Autodesk Inventor part; units mm, degrees
ref_plane "YZ Plane" through (0, 0, 0) normal (1, 0, 0) x (0, 1, 0)
ref_plane "XZ Plane" through (0, 0, 0) normal (0, 1, 0) x (-1, 0, 0)
ref_plane "XY Plane" through (0, 0, 0) normal (0, 0, 1) x (1, 0, 0)
sketch "Sketch1" plane through (0, 0, 0) normal (0, 0, 1) x (1, 0, 0)
  line L0 (0, 0) -> (15.24, 0)
  line L1 (15.24, 0) -> (15.24, 25.4)
  line L2 (15.24, 25.4) -> (0, 25.4)
  line L3 (0, 25.4) -> (0, 0)
  dimension "d0" = 15.24
  dimension "d1" = 25.4
extrude "Extrusion1" add sketch "Sketch1" along normal blind 3.175
sketch "Sketch2" plane through (0, 0, 3.175) normal (0, 0, 1) x (1, 0, 0)
  line L0 (15.24, 25.4) -> (0, 25.4)
  line L1 (0, 25.4) -> (4.826, 25.4)
  line L2 (4.826, 25.4) -> (4.826, 22.86)
  line L3 (4.826, 22.86) -> (0, 22.86)
  line L4 (0, 22.86) -> (0, 25.4)
  line L5 (15.24, 25.4) -> (0, 25.4)
  line L6 (15.24, 25.4) -> (10.414, 25.4)
  line L7 (10.414, 25.4) -> (10.414, 22.86)
  line L8 (10.414, 22.86) -> (15.24, 22.86)
  line L9 (15.24, 22.86) -> (15.24, 25.4)
  point P0 (0, 0)
  dimension "d4" = 4.826
  dimension "d5" = 2.54
  dimension "d6" = 4.826
extrude "Extrusion2" add sketch "Sketch2" along normal blind 10.16
chamfer "Chamfer1" distance 4.826 angle 45 2 edges at (4.826, 24.13, 13.335) (10.414, 24.13, 13.335)
fillet "Fillet1" radius 1.27 2 edges at (4.826, 24.13, 3.175) (10.414, 24.13, 3.175)
fillet "Fillet2" radius 3.175 2 edges at (15.24, 0, 1.5875) (0, 0, 1.5875)
properties part number "Cable managment."
Source: CAD feature listing. Evaluate the final solid. Frame: model axes, mm. A direction names the side the tool comes from. Give positions to 0.01 mm unless a question says otherwise; leave off trailing zeros. Write each loop counter-clockwise with the first axis right and the second up, starting at its lowest first coordinate (ties: lowest second). Pieces come first, ordered by that corner, then holes. Notation, with made-up numbers: M 56.25,29.25 L 106.25,29.25 A26 ccw 106.25,66.25 Z; hole C 69,-24.75 d10. An arc over 180 degrees is marked long. Return JSON: item names as keys, results as strings. Group by question number.
1) Ray query, L1, parallel to Z at x = 10.75, y = 3 (3 decimals); L2, parallel to Y at x = 4.5, z = 5. Return the intervals inside material, ascending.
2) Set-up query: faces 4 (the face through (8, 25.4, 2)), 5 (the face through (13, 22.86, 7)), 6 (the face through (4.826, 24, 6)). Return all of +Z, -Z, +X, -X, +Y, -Y with unobstructed straight access to the full face (end or side cutting, diameter ignored); none if empty.
3) Cut plane B-B, the plane x = 6.75. Output: boundary loops of the cut face in (y, z) (3 decimals).
4) Draft query along X for faces 1 (the face through (2, 22.86, 7)), 2 (the face through (5.188, 24.112, 3.557)), 3 (the face through (14.29, 0.91, 1.61)). Return one class per face: released by +X, released by -X, zero draft, split by the parting line, or undercut.
5) Cut plane C-C, the plane z = 9. Output: boundary loops of the cut face in (x, y), then the cut area to 3 significant figures.
6) First-contact query: pin 1 Ø4 at (y, z) = (3.5, 3.5) entering from -X; pin 2 Ø1 at (x, z) = (8.5, 7.5) entering from -Y; pin 3 Ø5 at (x, y) = (3, 3) entering from +Z (3 decimals); pin 4 Ø3 at (x, z) = (4, 6) entering from -Y. Flat tips, straight axial feed; report the tip coordinate or a pass-through.
7) Cut plane A-A, the plane z = 6. Output: boundary loops of the cut face in (x, y).
8) Cut plane D-D, the plane y = 5.5. Output: boundary loops of the cut face in (x, z) (3 decimals), then the cut area to 3 significant figures.
Data:
{
 "1": {"L1": "z = 0 to 3.175", "L2": "y = 22.86 to 25.4"},
 "2": {"face 4": "+Z, -Z, +X, -X, +Y", "face 5": "+Z, +X, -X, -Y", "face 6": "+Z, +Y, -Y"},
 "3": {"outline": "M 0,0 L 25.4,0 L 25.4,3.175 L 0,3.175 Z"},
 "4": {"face 1": "zero draft", "face 2": "undercut", "face 3": "released by +X"},
 "5": {"outline": "M 0,22.86 L 4.34,22.86 L 4.34,25.4 L 0,25.4 Z; M 10.9,22.86 L 15.24,22.86 L 15.24,25.4 L 10.9,25.4 Z", "area": "22.0 mm²"},
 "6": {"pin 1": "stops at x = 0", "pin 2": "passes through", "pin 3": "stops at z = 3.175", "pin 4": "stops at y = 22.86"},
 "7": {"outline": "M 0,22.86 L 4.83,22.86 L 4.83,25.4 L 0,25.4 Z; M 10.41,22.86 L 15.24,22.86 L 15.24,25.4 L 10.41,25.4 Z"},
 "8": {"outline": "M 0,0 L 15.24,0 L 15.24,3.175 L 0,3.175 Z", "area": "48.4 mm²"}
}
